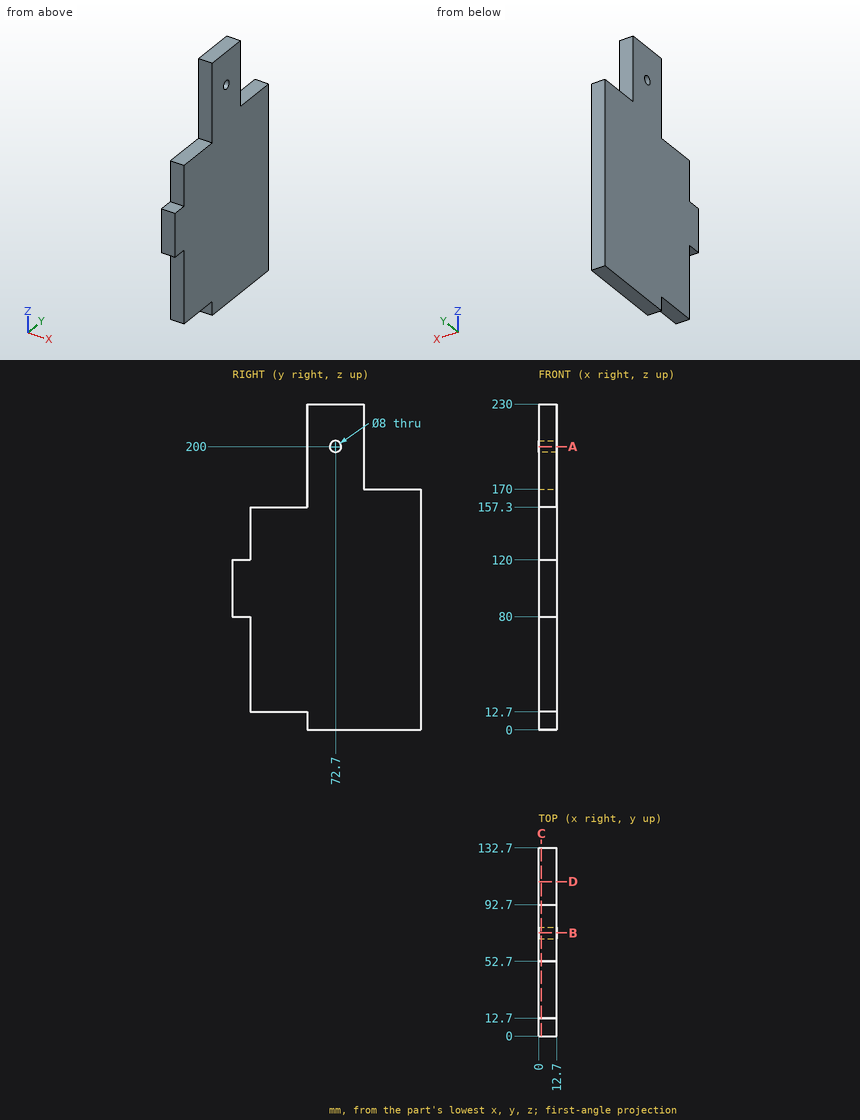
Here's the drawing with two shaded views (mm, measured from the low corner). I have some questions. Round coordinates to 2 decimals unless told otherwise and drop trailing zeros. Loops run counter-clockwise (first coordinate to the right, second up) from the corner with the lowest first, then second, coordinate; pieces in that order, holes last.
Item 1: Suppose I cut it at B-B, the plane y = 72.7. Write out the boundary of the cut face in (x, z), then the cut area to 3 significant figures.
Item 2: Suppose I cut it at C-C, the plane x = 2. Write out the boundary of the cut face in (y, z), then the cut area to 3 significant figures.
Item 3: Will these pins go through, and if not, where does the flat tip stop? pin 1 Ø6.5 at (x, z) = (4.5, 193.5) entering from -Y; pin 2 Ø8 at (y, z) = (97, 112.5) entering from -X; pin 3 Ø5 at (x, z) = (6.5, 194) entering from +Y; pin 4 Ø2 at (x, y) = (9.5, 111.5) entering from +Z.
Item 4: Suppose I cut it at A-A, the plane z = 200. Write out the boundary of the cut face in (x, y).
Item 5: Suppose I cut it at D-D, the plane y = 109. Write out the boundary of the cut face in (x, z).
Item 6: Please list where these lines run through material, in increasing order: L1, parallel to Y at x = 3.25, z = 200; L2, parallel to Z at x = 9.25, y = 72.7; L3, parallel to Z at x = 6.25, y = 96.
Reported:
1. outline: (0, 0) - (12.7, 0) - (12.7, 196) - (0, 196) - close; (0, 204) - (12.7, 204) - (12.7, 230) - (0, 230) - close
1. area: 2,820 mm2
2. outline: (0, 80) - (12.7, 80) - (12.7, 12.7) - (52.7, 12.7) - (52.7, 0) - (132.7, 0) - (132.7, 170) - (92.7, 170) - (92.7, 230) - (52.7, 230) - (52.7, 157.3) - (12.7, 157.3) - (12.7, 120) - (0, 120) - close; hole circle Ø8 at (72.7, 200)
2. area: 22,200 mm2
3. pin 1: stops at y = 52.7
3. pin 2: stops at x = 0
3. pin 3: stops at y = 92.7
3. pin 4: stops at z = 170
4. outline: (0, 52.7) - (12.7, 52.7) - (12.7, 68.7) - (0, 68.7) - close; (0, 76.7) - (12.7, 76.7) - (12.7, 92.7) - (0, 92.7) - close
5. outline: (0, 0) - (12.7, 0) - (12.7, 170) - (0, 170) - close
6. L1: y = 52.7 to 68.7, 76.7 to 92.7
6. L2: z = 0 to 196, 204 to 230
6. L3: z = 0 to 170
